```python
from build123d import *

# Parameters (mm, degrees)
F0_W           = 80
F0_H           = 43
F1_DEPTH       = 25
F2_W           = 3
F2_H           = 27
F3_DEPTH       = 80.001
F4_R           = 2.5
F5_DEPTH       = 25.001
F6_D           = 4
F6_CSINK_D     = 9.2
F6_CSINK_ANGLE = 90
F7_D           = 5
F7_CSINK_D     = 11.5
F7_CSINK_ANGLE = 90


with BuildPart() as f1:
    # F0 (on Front) → F1 (new body)
    with BuildSketch(Plane.XZ):
        Rectangle(F0_W, F0_H)
    extrude(amount=F1_DEPTH)

    # F2 (on face) → F3 (cut, through all)
    with BuildSketch(Plane.YZ.offset(40)):
        with Locations((-23.5, -8)):
            Rectangle(F2_W, F2_H)
    extrude(amount=-F3_DEPTH, mode=Mode.SUBTRACT)

    # F4 (on face) → F5 (cut, through all)
    with BuildSketch(Plane(origin=(0, 0, 0), x_dir=(-1, 0, 0), z_dir=(0, 1, 0))):
        with Locations((-8.1, -8)):
            Circle(F4_R)
        with Locations((8.1, -8)):
            Circle(F4_R)
    extrude(amount=-F5_DEPTH, mode=Mode.SUBTRACT)

    # F6 (through all)
    with Locations(Plane(origin=(0, 0, 0), x_dir=(-1, 0, 0), z_dir=(0, 1, 0))):
        with Locations((-15.05, 10.55), (15.05, 10.55)):
            CounterSinkHole(F6_D / 2, F6_CSINK_D / 2, counter_sink_angle=F6_CSINK_ANGLE)

    # F7 (through all)
    with Locations(Plane(origin=(0, 0, 0), x_dir=(-1, 0, 0), z_dir=(0, 1, 0))):
        with Locations((-22.25, -8), (22.25, -8)):
            CounterSinkHole(F7_D / 2, F7_CSINK_D / 2, counter_sink_angle=F7_CSINK_ANGLE)


solid = f1.part
```
Work out the finished part from the listing and answer in its coordinate system (mm). A direction names the side the tool comes from. Give positions to 0.01 mm unless a question says otherwise; leave off trailing zeros. Loops run counter-clockwise (first coordinate to the right, second up) from the corner with the lowest first, then second, coordinate; pieces in that order, holes last. Notation, with made-up numbers: M -7.75,58.5 L 40.25,58.5 A21 ccw 40.25,89.5 Z; hole C 27.25,34 d5. An arc over 180 degrees is marked long. One line per item, written item: value. Start each with the question number.
1. Find section D-D (z = 10.55). Give the vertices of the cut face in (x, y), and give its area (3 significant figures).
2. Find section C-C (y = -23). Give the vertices of the cut face in (x, z), and give its area (3 significant figures).
3. Each of these flat-tipped pins is pushed along its axis until it touches: P1, Ø6.5, axis at x = 22.25, z = -8, coming from the +Y side; P2, Ø8, axis at x = -22.25, z = -8, coming from the -Y side; P3, Ø3, axis at x = -15.05, z = 10.55, coming from the -Y side; P4, Ø0.9, axis at x = 10.5, y = -23, coming from the -Z side. Where does it stop, or does it pass through?
4. Determine the mould class of faces 3 (the face through (-1, -12, 21.5)), 4 (the face through (40, -12, 0)), 5 (the face through (-6.1, -10.8, -9.5)) for opening direction Z: released by +Z, released by -Z, zero draft, split by the parting line, or undercut.
5. Which of the six approach directions +Z, -Z, +X, -X, +Y, -Y give full straight-line access (tool end or side, diameter ignored) to faces 1 (the face through (1, -24, 5.5)), 2 (the face through (-19.795, -3.092, -9.018))?
6. Find the intervals of material crossed by probe 1 along X at (y, z) = (-13.25, 10.55); probe 2 along Z at (x, y) = (22.25, -13.5); probe 3 along Z at (x, y) = (-15.05, -20), in increasing order.
7. Find section B-B (z = -8). Give the vertices of the cut face in (x, y).
8. Find section A-A (x = -15.05). Give the vertices of the cut face in (y, z), and give its area (3 significant figures).
Reported:
1. outline: M -40,-25 L -17.05,-25 L -17.05,-2.6 L -19.65,0 L -40,0 Z; M -13.05,-25 L 13.05,-25 L 13.05,-2.6 L 10.45,0 L -10.45,0 L -13.05,-2.6 Z; M 17.05,-25 L 40,-25 L 40,0 L 19.65,0 L 17.05,-2.6 Z
1. area: 1,790 mm²
2. outline: M -40,5.5 L 40,5.5 L 40,21.5 L -40,21.5 Z; hole C -15.05,10.55 d4; hole C 15.05,10.55 d4
2. area: 1,250 mm²
3. P1: stops at y = -2.5
3. P2: stops at y = -22
3. P3: passes through
3. P4: stops at z = 5.5
4. face 3: released by +Z
4. face 4: zero draft
4. face 5: undercut
5. face 1: -Z, +X, -X, -Y
5. face 2: +Y
6. probe 1: x = -40 to -17.05, -13.05 to 13.05, 17.05 to 40
6. probe 2: z = -21.5 to -10.5, -5.5 to 21.5
6. probe 3: z = -21.5 to 8.55, 12.55 to 21.5
7. outline: M -40,-22 L -24.75,-22 L -24.75,-3.25 L -28,0 L -40,0 Z; M -19.75,-22 L -10.6,-22 L -10.6,0 L -16.5,0 L -19.75,-3.25 Z; M -5.6,-22 L 5.6,-22 L 5.6,0 L -5.6,0 Z; M 10.6,-22 L 19.75,-22 L 19.75,-3.25 L 16.5,0 L 10.6,0 Z; M 24.75,-22 L 40,-22 L 40,0 L 28,0 L 24.75,-3.25 Z
8. outline: M -25,5.5 L -22,5.5 L -22,-21.5 L 0,-21.5 L 0,5.95 L -2.6,8.55 L -25,8.55 Z; M -25,12.55 L -2.6,12.55 L 0,15.15 L 0,21.5 L -25,21.5 Z
8. area: 887 mm²
